Could you check a few things on this drawing? It's one solid part, dimensions in mm from its lowest x, y, z. A direction names the side the tool comes from. Coordinates: 2 decimals unless noted, no trailing zeros. Loops run counter-clockwise (first coordinate to the right, second up) from the corner with the lowest first, then second, coordinate; pieces in that order, holes last. Notation, with made-up numbers: (-26.5, 70) -> (-4.5, 70) arc R36 cw to (-4.5, 109) -> close; hole circle Ø7 at (50.5, 59.5). An arc over 180 degrees is marked (long way). One line per question, with ' | ' between items. Start each with the question number.
(1) If I drill on line 1 along Z through (x, y) = (9.5, 5.5); line 2 along Y through (x, z) = (8, 2); line 3 along Y through (x, z) = (5.5, 1.75), over which ranges is the centre line in solid material (lowest first)?
(2) Suppose I cut it at C-C (z = 6.75). Please give me the cut outline in (x, y), plus the area to 3 significant figures.
(3) Suppose I cut it at D-D (z = 1.5). Please give me the cut outline in (x, y).
(4) Suppose I cut it at A-A (x = 8.2). Please give me the cut outline in (y, z).
(5) Which directions (+Z, -Z, +X, -X, +Y, -Y) give clear straight access to the entire face, cutting with the end or side of a thin tool? Please do the marked faces 1 and 2.
(6) I'm going to push a flat-ended pin straight in: pin 1 Ø1 at (x, y) = (14, 6) entering from +Z. Where does the tip first touch, or does it pass through?
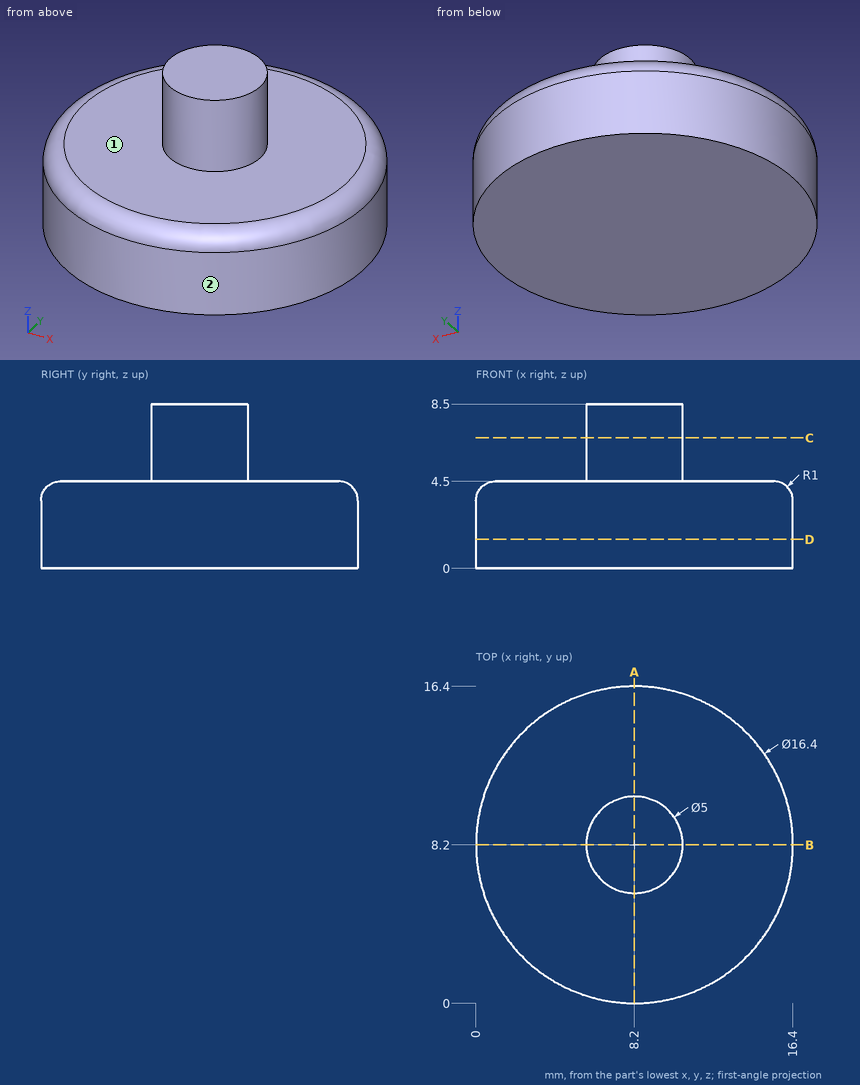
Checks:
1) line 1: z = 0 to 4.5 | line 2: y = 0 to 16.4 | line 3: y = 0.46 to 15.94
2) outline: circle Ø5 at (8.2, 8.2) | area: 19.6 mm^2
3) outline: circle Ø16.4 at (8.2, 8.2)
4) outline: (0, 0) -> (16.4, 0) -> (16.4, 3.5) arc R1 ccw to (15.4, 4.5) -> (10.7, 4.5) -> (10.7, 8.5) -> (5.7, 8.5) -> (5.7, 4.5) -> (1, 4.5) arc R1 ccw to (0, 3.5) -> close
5) face 1: +Z | face 2: +Z, -Z
6) pin 1: stops at z = 4.5
